Work out the finished part from the listing and answer in its coordinate system (mm). Give positions to 0.01 mm unless a question says otherwise; leave off trailing zeros. Write each loop counter-clockwise with the first axis right and the second up, starting at its lowest first coordinate (ties: lowest second). Pieces come first, ordered by that corner, then holes.
1) Given pin 1 Ø5 at (y, z) = (-7.5, 160.5) entering from -X; pin 2 Ø3 at (x, y) = (33, -9.5) entering from +Z; pin 3 Ø1.5 at (x, y) = (23.5, 5) entering from +Z, each flat-ended and moving along its own axis, determine where each tip first touches the part or whether it passes through.
2) Straight lines are drawn through the part: probe 1 along Y at (x, z) = (-36, 218.5); probe 2 along X at (y, z) = (24.5, 164.5); probe 3 along X at (y, z) = (1.5, 251). For each, find the intervals that lie inside material, in ascending order.
3) Find section A-A (z = 117). Determine the outline of the cut face in (x, y), plus the area to 3 significant figures.
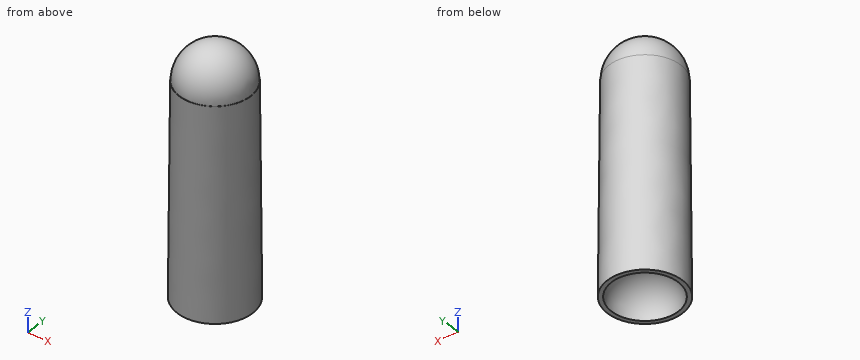
```python
from build123d import *

# Parameters (mm, degrees)
SKETCH1_R           = 44.55
BOSS_EXTRUDE1_DEPTH = 250
BOSS_EXTRUDE1_TAPER = 0.5


with BuildPart() as part:
    # Sketch1 → Boss-Extrude1 (new body)
    with BuildSketch(Plane.XY):
        Circle(SKETCH1_R)
    extrude(amount=BOSS_EXTRUDE1_DEPTH, taper=BOSS_EXTRUDE1_TAPER)

    # Sketch2 → Cut-Revolve1 (revolve, cut)
    with BuildSketch(Plane(origin=(0, 0, 0), x_dir=(-1, 0, 0), z_dir=(0, 0, -1))):
        with BuildLine():
            Line((0, 39.55), (0, -39.55))
            ThreePointArc((0, -39.55), (39.55, 0), (0, 39.55))
        make_face()
    revolve(axis=Axis((0, 39.55, 0), (0, -1, 0)), mode=Mode.SUBTRACT)

    # Sketch3 → Revolve1 (revolve)
    with BuildSketch(Plane.XY.offset(250)):
        with BuildLine():
            Line((0, 42.106477019), (0, -42.106477019))
            ThreePointArc((0, -42.106477019), (-42.106477019, 0), (0, 42.106477019))
        make_face()
    revolve(axis=Axis((0, 42.106477019, 250), (0, -1, 0)))


solid = part.part
```
Results:
1. pin 1: stops at x = -42.86
1. pin 2: stops at z = 276.35
1. pin 3: stops at z = 285.09
2. probe 1: y = -22.86 to 22.86
2. probe 2: x = -35.48 to 35.48
2. probe 3: x = -42.07 to 42.07
3. outline: circle Ø87.06 at (0, 0)
3. area: 5,950 mm2
